Source: CAD feature listing. Evaluate the final solid. Frame: model axes, mm. A direction names the side the tool comes from. Give positions to 0.01 mm unless a question says otherwise; leave off trailing zeros. Order: outer loops, then holes, each group sorted by start corner. A loop starts at its lowest first (then second) coordinate and runs counter-clockwise, first axis right, second up. Notation, with made-up numbers: M 38,37.5 L 51,37.5 A13 ccw 51,52.5 Z; hole C -16.75,32 d8. An arc over 180 degrees is marked long. Use CSV: the item, a comma, the result in double quotes. Start each with the question number.
1. Section query A-A, the plane z = 34.5. Return the cut outline in (x, y), plus the area to 3 significant figures.
2. Reachability of faces 1 (the cylindrical face through (-19.95, -30.46, 33.1)), 2 (the cylindrical face through (-24.577, 0.363, 23.504)) from +Z, -Z, +X, -X, +Y, -Y: full face, straight path, thin tool, end or side. Return the list, or none.
3. Section query D-D, the plane y = 0. Return the cut outline in (x, z), plus the area to 3 significant figures.
4. Pin query (flat end, axial travel): P1, Ø5, axis at x = 8, y = -12.5, coming from the +Z side; P2, Ø15, axis at y = -1, z = 34, coming from the -X side; P3, Ø4, axis at x = -22, y = 30, coming from the +Z side; P4, Ø3.5, axis at x = -22, y = -30, coming from the +Z side. Return the tip coordinate at first contact, or that it passes through.
5. Line query: line 1 along X through (y, z) = (-30, 36); line 2 along X through (y, z) = (8, 10.5); line 3 along X through (y, z) = (16, 32.5). Output: solid intervals per line, ascending. Write a range as [from, to].
6. Mould query, pull axis Y, two halves, no side actions, for faces 3 (the flat face through (-19, 4.2, 23.85)), 4 (the flat face through (30, -1, 20)), 5 (the flat face through (0, -40, 20)), 6 (the cylindrical face through (-19.95, 30.46, 33.1)). Classes: released by +Y, released by -Y, zero draft, split by the parting line, or undercut.
7. Section query C-C, the plane z = 14.5. Return the cut outline in (x, y).
8. Section query B-B, the plane x = 25.5. Return the cut outline in (y, z).
from build123d import *

# Parameters (mm, degrees)
SCHIZZO1_W                   = 60
SCHIZZO1_H                   = 80
ESTRUSIONE_ESTRUSIONE1_DEPTH = 40
SCHIZZO3_R                   = 16.5
TAGLIO_ESTRUSIONE1_DEPTH     = 11
SCHIZZO4_R                   = 18.5
TAGLIO_ESTRUSIONE2_DEPTH     = 12
SCHIZZO5_R                   = 34
TAGLIO_ESTRUSIONE3_DEPTH     = 20
SCHIZZO6_R                   = 18.5
TAGLIO_ESTRUSIONE4_DEPTH     = 9
SCHIZZO7_R                   = 16.5
TAGLIO_ESTRUSIONE5_DEPTH     = 8


with BuildPart() as part:
    # Schizzo1 → Estrusione-Estrusione1 (new body)
    with BuildSketch(Plane.XY):
        Rectangle(SCHIZZO1_W, SCHIZZO1_H)
    extrude(amount=ESTRUSIONE_ESTRUSIONE1_DEPTH)

    # Schizzo3 → Taglio-Estrusione1 (cut)
    with BuildSketch(Plane.ZY.offset(30)):
        with Locations((40, 0)):
            Circle(SCHIZZO3_R)
    extrude(amount=-TAGLIO_ESTRUSIONE1_DEPTH, mode=Mode.SUBTRACT)

    # Schizzo4 → Taglio-Estrusione2 (cut)
    with BuildSketch(Plane.ZY.offset(19)):
        with Locations((40, 0)):
            Circle(SCHIZZO4_R)
    extrude(amount=-TAGLIO_ESTRUSIONE2_DEPTH, mode=Mode.SUBTRACT)

    # Schizzo5 → Taglio-Estrusione3 (cut)
    with BuildSketch(Plane.ZY.offset(7)):
        with Locations((40, 0)):
            Circle(SCHIZZO5_R)
    extrude(amount=-TAGLIO_ESTRUSIONE3_DEPTH, mode=Mode.SUBTRACT)

    # Schizzo6 → Taglio-Estrusione4 (cut)
    with BuildSketch(Plane.ZY.offset(-13)):
        with Locations((40, 0)):
            Circle(SCHIZZO6_R)
    extrude(amount=-TAGLIO_ESTRUSIONE4_DEPTH, mode=Mode.SUBTRACT)

    # Schizzo7 → Taglio-Estrusione5 (cut)
    with BuildSketch(Plane.ZY.offset(-22)):
        with Locations((40, 0)):
            Circle(SCHIZZO7_R)
    extrude(amount=-TAGLIO_ESTRUSIONE5_DEPTH, mode=Mode.SUBTRACT)

    # Schizzo9 → Foro filettato M5-1 (revolve, cut)
    with BuildSketch(Plane(origin=(-22, 30, 40), x_dir=(0, -1, 0), z_dir=(1, 0, 0))):
        Polygon((0, 0), (0, 15.2618073), (2.1, 14), (2.1, 0), align=None)
    foro_filettato_m5_1 = revolve(axis=Axis((-22, 30, 46.35), (0, 0, -1)), mode=Mode.SUBTRACT)

    # Specchia1: Foro filettato M5-1 across plane
    add(foro_filettato_m5_1.mirror(Plane.ZX), mode=Mode.SUBTRACT)

    # Specchia2: Foro filettato M5-1 across plane
    add(foro_filettato_m5_1.mirror(Plane(origin=(0, 0, 0), x_dir=(0, 0, 1), z_dir=(1, 0, 0))), mode=Mode.SUBTRACT)

    # Specchia2 copy 1 sketch → Specchia2 copy 1 (revolve, cut)
    with BuildSketch(Plane(origin=(22, -30, 40), x_dir=(0, 1, 0), z_dir=(-1, 0, 0))):
        Polygon((0, 0), (0, 15.2618073), (2.1, 14), (2.1, 0), align=None)
    revolve(axis=Axis((22, -30, 46.35), (0, 0, -1)), mode=Mode.SUBTRACT)


solid = part.part
Result set:
1,outline,"M -30,-40 L 30,-40 L 30,-15.56 L 22,-15.56 L 22,-17.66 L 13,-17.66 L 13,-33.55 L -7,-33.55 L -7,-17.66 L -19,-17.66 L -19,-15.56 L -30,-15.56 Z; M -30,15.56 L -19,15.56 L -19,17.66 L -7,17.66 L -7,33.55 L 13,33.55 L 13,17.66 L 22,17.66 L 22,15.56 L 30,15.56 L 30,40 L -30,40 Z; hole C -22,-30 d4.2; hole C -22,30 d4.2; hole C 22,-30 d4.2; hole C 22,30 d4.2"
1,area,"2,070 mm2"
2,face 1,"+Z"
2,face 2,"+Z, +X, -X"
3,outline,"M -30,0 L 30,0 L 30,23.5 L 22,23.5 L 22,21.5 L 13,21.5 L 13,6 L -7,6 L -7,21.5 L -19,21.5 L -19,23.5 L -30,23.5 Z"
3,area,"1,020 mm2"
4,P1,"z = 9.49"
4,P2,"through"
4,P3,"z = 25.94"
4,P4,"z = 25.79"
5,line 1,"[-30, -24.1], [-19.9, -7], [13, 19.9], [24.1, 30]"
5,line 2,"[-30, -7], [13, 30]"
5,line 3,"[-30, -19], [22, 30]"
6,face 3,"undercut"
6,face 4,"zero draft"
6,face 5,"released by -Y"
6,face 6,"undercut"
7,outline,"M -30,-40 L 30,-40 L 30,40 L -30,40 Z; hole M -7,-22.49 L 13,-22.49 L 13,22.49 L -7,22.49 Z"
8,outline,"M -40,0 L 40,0 L 40,40 L 16.5,40 A16.5 cw -16.5,40 L -40,40 Z"
